from build123d import *

# Parameters (mm, degrees)
IZIM2_W                     = 2.48
IZIM2_H                     = 6.762592592
Y_KSEKLIK_EKSTR_ZYON2_DEPTH = 5.86
Y_KSEKLIK_EKSTR_ZYON3_DEPTH = 0.4


# Read off the part's stored shape, not the designer's step: Döndür1
with BuildPart() as part:
    # Çizim2 → Yükseklik-Ekstrüzyon2 (new body)
    with BuildSketch(Plane(origin=(0, 0, 0), x_dir=(0, 0, -1), z_dir=(1, 0, 0))):
        Rectangle(IZIM2_W, IZIM2_H)
    extrude(amount=-Y_KSEKLIK_EKSTR_ZYON2_DEPTH)

    # Döndür1 outline → Döndür1 (revolve)
    with BuildSketch(Plane(origin=(-2.93, 0, 1.24), x_dir=(1, 0, 0), z_dir=(0, 0, 1))):
        with BuildLine():
            Line((0, 2.378703704), (0, -3.381296296))
            Line((0, -3.381296296), (1.94, -3.381296296))
            Line((1.94, -3.381296296), (1.94, 0.438703704))
            ThreePointArc((1.94, 0.438703704), (1.371787155, 1.810490859), (0, 2.378703704))
        make_face()
    revolve(axis=Axis((-2.93, 0, 1.24), (0, 1, 0)))

    # Çizim6 → Yükseklik-Ekstrüzyon3 (add)
    with BuildSketch(Plane(origin=(0, 0, -0.74), x_dir=(-1, 0, 0), z_dir=(0, 0, -1))):
        with BuildLine():
            Line((2.43, -3.381296296), (2.43, -4.381296296))
            ThreePointArc((2.43, -4.381296296), (2.459289322, -4.452006974), (2.53, -4.481296296))
            Line((2.53, -4.481296296), (2.68, -4.481296296))
            Line((2.68, -4.481296296), (2.68, -5.231296296))
            Line((2.68, -5.231296296), (2.58, -5.231296296))
            Line((2.58, -5.231296296), (2.58, -5.981296296))
            Line((2.58, -5.981296296), (2.68, -5.981296296))
            Line((2.68, -5.981296296), (2.68, -26.481296296))
            Line((2.68, -26.481296296), (3.18, -26.481296296))
            Line((3.18, -26.481296296), (3.18, -5.981296296))
            Line((3.18, -5.981296296), (3.28, -5.981296296))
            Line((3.28, -5.981296296), (3.28, -5.231296296))
            Line((3.28, -5.231296296), (3.18, -5.231296296))
            Line((3.18, -5.231296296), (3.18, -4.481296296))
            Line((3.18, -4.481296296), (3.33, -4.481296296))
            ThreePointArc((3.33, -4.481296296), (3.400710678, -4.452006974), (3.43, -4.381296296))
            Line((3.43, -4.381296296), (3.43, -3.381296296))
            Line((3.43, -3.381296296), (2.43, -3.381296296))
        make_face()
        Polygon((5.22, -4.481296296), (5.22, -5.231296296), (5.12, -5.231296296), (5.12, -5.981296296), (5.22, -5.981296296), (5.22, -26.481296296), (5.72, -26.481296296), (5.72, -5.981296296), (5.82, -5.981296296), (5.82, -5.231296296), (5.72, -5.231296296), (5.72, -4.481296296), (5.72, -3.981296296), (5.22, -3.981296296), (5.22, -3.381296296), (4.86, -3.381296296), (4.86, -4.481296296), align=None)
        Polygon((0.14, -4.481296296), (0.14, -5.231296296), (0.04, -5.231296296), (0.04, -5.981296296), (0.14, -5.981296296), (0.14, -26.481296296), (0.64, -26.481296296), (0.64, -5.981296296), (0.74, -5.981296296), (0.74, -5.231296296), (0.64, -5.231296296), (0.64, -4.481296296), (1, -4.481296296), (1, -3.381296296), (0.64, -3.381296296), (0.64, -3.981296296), (0.14, -3.981296296), align=None)
    extrude(amount=-Y_KSEKLIK_EKSTR_ZYON3_DEPTH)


solid = part.part
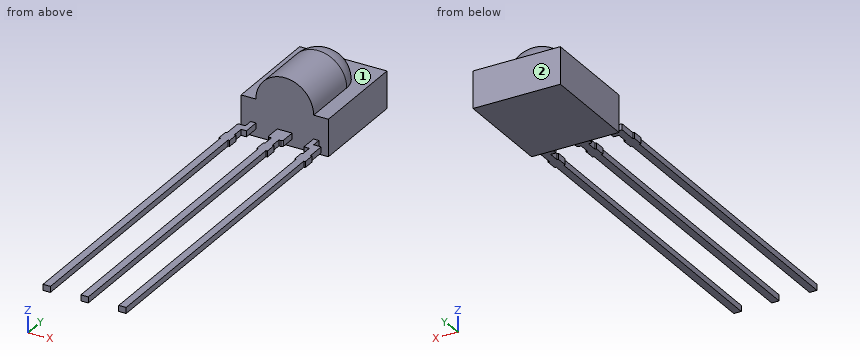
Geometry: final body of the model. Coordinates: model frame, mm. Face numbers are marked on the shaded views. A direction names the side the tool comes from. Round coordinates to 2 decimals unless told otherwise and drop trailing zeros. Loops run counter-clockwise (first coordinate to the right, second up) from the corner with the lowest first, then second, coordinate; pieces in that order, holes last. Notation, with made-up numbers: (62.25, 7.5) -> (79.25, 7.5) arc R9 ccw to (79.25, 12.5) -> close; hole circle Ø10 at (-1.75, 87). An arc over 180 degrees is marked (long way). One line per question, with ' | ' between items. Start each with the question number.
1. Line query: line 1 along Y through (x, z) = (-5.3, 1.05); line 2 along Y through (x, z) = (-0.3, -0.4); line 3 along Z through (x, y) = (-0.85, -1.5). Output: solid intervals per line, ascending. Write a range as [from, to].
2. Section C-C on y = -2.75. Output: boundary loops of the cut face in (x, z).
3. Section A-A on y = -21. Output: boundary loops of the cut face in (x, z), and give its area (3 significant figures).
4. Contact query for flat-ended pins moving along their axis: pin 1 (2 mm diameter, centred on x = -3, z = 1.5, fed in from -Y); pin 2 (3 mm diameter, centred on x = -3, y = -18.5, fed in from -Z); pin 3 (2 mm diameter, centred on x = -4, z = 2.5, fed in from +Y). Output: stop coordinate, or through.
5. Section D-D on z = 0.1. Output: boundary loops of the cut face in (x, y), and give its area (3 significant figures).
6. Set-up query: the marked faces 1 and 2. Return all of +Z, -Z, +X, -X, +Y, -Y with unobstructed straight access to the full face (end or side cutting, diameter ignored); none if empty.
7. Section B-B on x = -2.93. Output: boundary loops of the cut face in (y, z), and give its area (3 significant figures).
Returned:
1) line 1: y = [-3.38, 3.38] | line 2: y = [-26.48, -3.98], [-3.38, 3.38] | line 3: z = [-1.24, 1.24]
2) outline: (-5.86, -1.24) -> (0, -1.24) -> (0, 1.24) -> (-0.99, 1.24) arc R1.94 ccw to (-4.87, 1.24) -> (-5.86, 1.24) -> close
3) outline: (-5.72, -0.74) -> (-5.22, -0.74) -> (-5.22, -0.34) -> (-5.72, -0.34) -> close; (-3.18, -0.74) -> (-2.68, -0.74) -> (-2.68, -0.34) -> (-3.18, -0.34) -> close; (-0.64, -0.74) -> (-0.14, -0.74) -> (-0.14, -0.34) -> (-0.64, -0.34) -> close | area: 0.600 mm2
4) pin 1: stops at y = -3.38 | pin 2: stops at z = -0.74 | pin 3: stops at y = 2.27
5) outline: (-5.86, -3.38) -> (0, -3.38) -> (0, 3.38) -> (-5.86, 3.38) -> close | area: 39.6 mm2
6) face 1: +Z, +Y | face 2: +Z, -Z, +X, -X, +Y
7) outline: (-26.48, -0.74) -> (-3.38, -0.74) -> (-3.38, -1.24) -> (3.38, -1.24) -> (3.38, 1.24) -> (2.38, 1.24) arc R1.94 ccw to (0.44, 3.18) -> (-3.38, 3.18) -> (-3.38, -0.34) -> (-26.48, -0.34) -> close | area: 36.4 mm2
